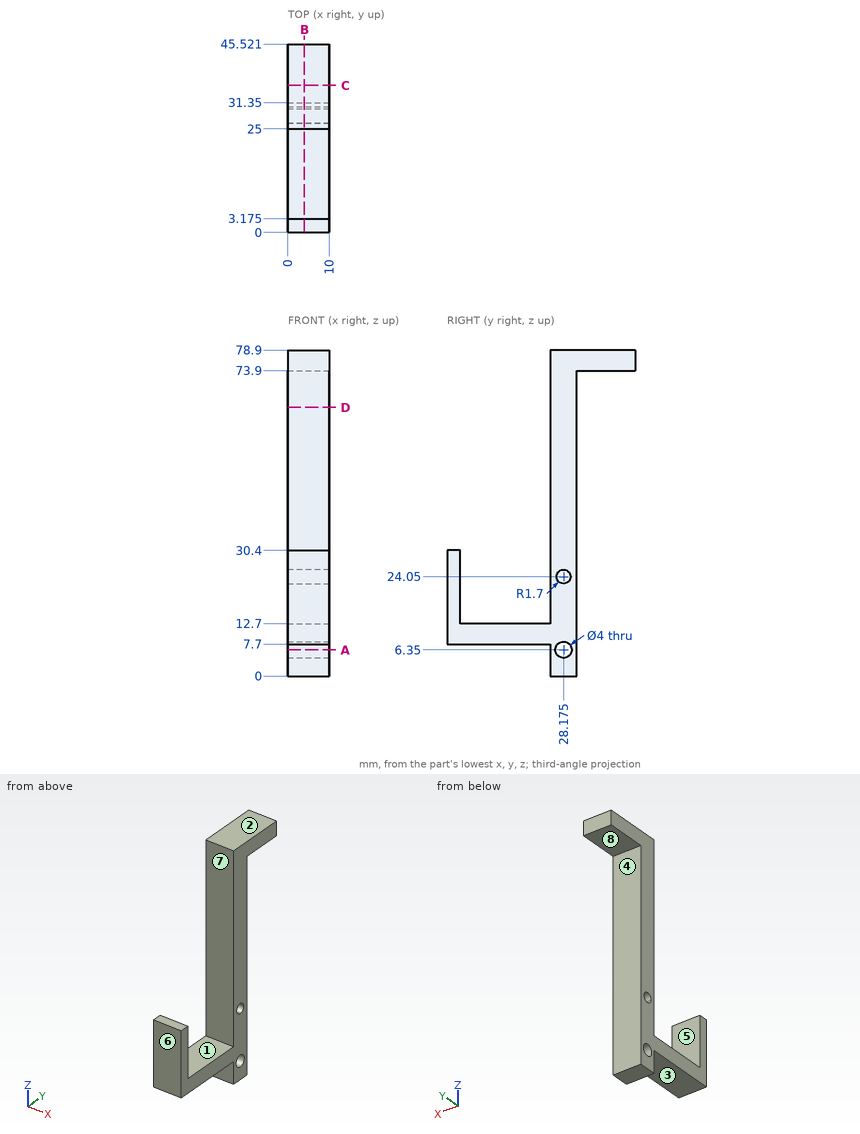
Can you work these out from the drawing? Everything is in mm from the part's minimum corner. A direction names the side the tool comes from. Coordinates: 2 decimals unless noted, no trailing zeros. Write each loop counter-clockwise with the first axis right and the second up, starting at its lowest first coordinate (ties: lowest second). Pieces come first, ordered by that corner, then holes. Notation, with made-up numbers: (-13, 57.25) -> (0, 57.25) arc R22 ccw to (0, 68.25) -> close; hole circle Ø9 at (21, 39). An arc over 180 degrees is marked (long way). Write each question's results on one line, items separated by ' | '. Start each with the question number.
Q1. Imagine slicing it at A-A (z = 6.35). Write out the boundary of the cut face in (x, y) (3 decimals), then the cut area to 3 significant figures.
Q2. On a 3-axis mill with a long thin cutter (end or side, diameter ignored), from which of +Z, -Z, +X, -X, +Y, -Y can I reach the whole of each face in a straight line? I mean the marked faces 1, 2, 3 and 4. Say none if no direction works.
Q3. Imagine slicing it at D-D (z = 65). Write out the boundary of the cut face in (x, y), then the cut area to 3 significant figures.
Q4. Imagine slicing it at B-B (x = 4). Write out the boundary of the cut face in (y, z) (3 decimals), then the cut area to 3 significant figures.
Q5. If I drill on probe 1 along Y at (x, z) = (1.75, 21) (3 decimals); probe 2 along Y at (x, z) = (2.75, 54); probe 3 along Y at (x, z) = (6.25, 6.5), over which ranges is the centre line in solid material (lowest first)?
Q6. Imagine slicing it at C-C (y = 35.5). Write out the boundary of the cut face in (x, z).
Q7. We'd pull the mould along Y, two halves only. Please class the marked faces 5, 6, 7 and 8: +Y half, -Y half, draft (parallel to the pull), parting line (faces both ways), or undercut.
Q8. I'm going to push flat-ended pins straight in: pin 1 (5 mm diameter, centred on x = 5.5, y = 10.5, fed in from +Z); pin 2 (3.5 mm diameter, centred on x = 5.5, y = 2, fed in from +Z); pin 3 (4 mm diameter, centred on x = 6, z = 3, fed in from -Y). Where does each tip first touch, or does it pass through?
Taken from the geometry:
1) outline: (0, 25) -> (10, 25) -> (10, 26.175) -> (0, 26.175) -> close; (0, 30.175) -> (10, 30.175) -> (10, 31.35) -> (0, 31.35) -> close | area: 23.5 mm^2
2) face 1: +Z, +X, -X | face 2: +Z, +X, -X, +Y, -Y | face 3: -Z, +X, -X, -Y | face 4: -Z, +X, -X, +Y
3) outline: (0, 25) -> (10, 25) -> (10, 31.35) -> (0, 31.35) -> close | area: 63.5 mm^2
4) outline: (0, 7.7) -> (25, 7.7) -> (25, 0) -> (31.35, 0) -> (31.35, 73.9) -> (45.521, 73.9) -> (45.521, 78.9) -> (25, 78.9) -> (25, 12.7) -> (3.175, 12.7) -> (3.175, 30.4) -> (0, 30.4) -> close; hole circle Ø4 at (28.175, 6.35); hole circle Ø3.4 at (28.175, 24.05) | area: 731 mm^2
5) probe 1: y = 0 to 3.175, 25 to 31.35 | probe 2: y = 25 to 31.35 | probe 3: y = 25 to 26.18, 30.17 to 31.35
6) outline: (0, 73.9) -> (10, 73.9) -> (10, 78.9) -> (0, 78.9) -> close
7) face 5: undercut | face 6: -Y half | face 7: undercut | face 8: draft
8) pin 1: stops at z = 12.7 | pin 2: stops at z = 30.4 | pin 3: stops at y = 25
